```python
from build123d import *

# Parameters (mm, degrees)
SKETCH_1_R               = 5.8
SKETCH_1_R_2             = 4.55
EXTRUDE_1_DEPTH          = 2.1
SKETCH_1_3_R             = 1.7
SKETCH_1_3_R_2           = 1
EXTRUDE_2_DEPTH          = 2.9
SKETCH_1_5_R             = 5.8
SKETCH_1_5_R_2           = 4.55
SKETCH_1_5_R_3           = 1.7
SKETCH_1_5_R_4           = 1
EXTRUDE_4_DEPTH          = 0.8
SKETCH_2_R               = 5.8
SKETCH_2_R_2             = 4.75
EXTRUDE_5_DEPTH          = 4.6
EXTRUDE_6_DEPTH          = 2
CUT_EXTRUDE_1_REACH      = 11.851
FILLET_1_R               = 0.2
FILLET_2_R               = 0.3
SKETCH_6_R               = 1.15
CUT_EXTRUDE_4_DEPTH      = 0.5
CUT_EXTRUDE_5_REACH      = 16.352
CUT_EXTRUDE_5_END_RADIUS = 4.75


with BuildPart() as part:
    # Sketch 1 → Extrude 1 (new body)
    with BuildSketch(Plane.XY):
        Circle(SKETCH_1_R)
        Circle(SKETCH_1_R_2, mode=Mode.SUBTRACT)
    extrude(amount=EXTRUDE_1_DEPTH)



with BuildPart() as body_2:
    # Sketch 1_3 → Extrude 2 (new body)
    with BuildSketch(Plane.XY):
        Circle(SKETCH_1_3_R)
        Circle(SKETCH_1_3_R_2, mode=Mode.SUBTRACT)
    extrude(amount=EXTRUDE_2_DEPTH)


with BuildPart() as part_1:
    add(part.part)

    add(body_2.part)  # Extrude 4 merges body 2
    # Sketch 1_5 → Extrude 4 (add)
    with BuildSketch(Plane.XY):
        Circle(SKETCH_1_5_R)
        Circle(SKETCH_1_5_R_2, mode=Mode.SUBTRACT)
        Circle(SKETCH_1_5_R_2)
        Circle(SKETCH_1_5_R_3, mode=Mode.SUBTRACT)
        Circle(SKETCH_1_5_R_3)
        Circle(SKETCH_1_5_R_4, mode=Mode.SUBTRACT)
    extrude(amount=-EXTRUDE_4_DEPTH)

    # Sketch 2 → Extrude 5 (add)
    with BuildSketch(Plane(origin=(0, 0, -0.8), x_dir=(-1, 0, 0), z_dir=(0, 0, -1))):
        Circle(SKETCH_2_R)
        Circle(SKETCH_2_R_2, mode=Mode.SUBTRACT)
    extrude(amount=EXTRUDE_5_DEPTH)

    # Sketch 3 → Extrude 6 (add)
    with BuildSketch(Plane(origin=(0, 0, -5.4), x_dir=(-1, 0, 0), z_dir=(0, 0, -1))):
        with BuildLine():
            Line((0, 5.8), (-2.93428015, 5.8))
            ThreePointArc((-2.93428015, 5.8), (-6.5, 0), (-2.93428015, -5.8))
            Line((-2.93428015, -5.8), (0, -5.8))
            ThreePointArc((0, -5.8), (-5.8, 0), (0, 5.8))
        make_face()
        with BuildLine():
            Line((2.93428015, 5.8), (0, 5.8))
            ThreePointArc((0, 5.8), (5.8, 0), (0, -5.8))
            Line((0, -5.8), (2.93428015, -5.8))
            ThreePointArc((2.93428015, -5.8), (6.5, 0), (2.93428015, 5.8))
        make_face()
    extrude(amount=-EXTRUDE_6_DEPTH)

    # Sketch 4 → Cut-Extrude 1 (cut, up to next)
    with BuildSketch(Plane(origin=(0, 0, -0.8), x_dir=(-1, 0, 0), z_dir=(0, 0, -1)), mode=Mode.PRIVATE) as cut_extrude_1_sk1:
        with BuildLine():
            Line((-0.7, -1.549193338), (-0.7, -2.19089023))
            ThreePointArc((-0.7, -2.19089023), (0, -2.3), (0.7, -2.19089023))
            Line((0.7, -2.19089023), (0.7, -1.549193338))
            ThreePointArc((0.7, -1.549193338), (0, -1.7), (-0.7, -1.549193338))
        make_face()
    cut_extrude_1_tool1 = extrude(cut_extrude_1_sk1.sketch, amount=-CUT_EXTRUDE_1_REACH, mode=Mode.PRIVATE) & part_1.part
    # Sketch 4 → Cut-Extrude 1 (cut, up to next)
    with BuildSketch(Plane(origin=(0, 0, -0.8), x_dir=(-1, 0, 0), z_dir=(0, 0, -1)), mode=Mode.PRIVATE) as cut_extrude_1_sk2:
        with BuildLine():
            ThreePointArc((0.7, 2.19089023), (0, 2.3), (-0.7, 2.19089023))
            Line((-0.7, 2.19089023), (-0.7, 1.549193338))
            ThreePointArc((-0.7, 1.549193338), (0, 1.7), (0.7, 1.549193338))
            Line((0.7, 1.549193338), (0.7, 2.19089023))
        make_face()
    cut_extrude_1_tool2 = extrude(cut_extrude_1_sk2.sketch, amount=-CUT_EXTRUDE_1_REACH, mode=Mode.PRIVATE) & part_1.part
    # Sketch 4 → Cut-Extrude 1 (cut, up to next)
    with BuildSketch(Plane(origin=(0, 0, -0.8), x_dir=(-1, 0, 0), z_dir=(0, 0, -1)), mode=Mode.PRIVATE) as cut_extrude_1_sk3:
        with BuildLine():
            ThreePointArc((-2.19089023, 0.7), (-2.3, 0), (-2.19089023, -0.7))
            Line((-2.19089023, -0.7), (-1.549193338, -0.7))
            ThreePointArc((-1.549193338, -0.7), (-1.7, 0), (-1.549193338, 0.7))
            Line((-1.549193338, 0.7), (-2.19089023, 0.7))
        make_face()
    cut_extrude_1_tool3 = extrude(cut_extrude_1_sk3.sketch, amount=-CUT_EXTRUDE_1_REACH, mode=Mode.PRIVATE) & part_1.part
    # Sketch 4 → Cut-Extrude 1 (cut, up to next)
    with BuildSketch(Plane(origin=(0, 0, -0.8), x_dir=(-1, 0, 0), z_dir=(0, 0, -1)), mode=Mode.PRIVATE) as cut_extrude_1_sk4:
        with BuildLine():
            Line((1.549193338, -0.7), (2.19089023, -0.7))
            ThreePointArc((2.19089023, -0.7), (2.272558858, -0.354226249), (2.3, 0))
            ThreePointArc((2.3, 0), (2.272558858, 0.354226249), (2.19089023, 0.7))
            Line((2.19089023, 0.7), (1.549193338, 0.7))
            ThreePointArc((1.549193338, 0.7), (1.661870734, 0.358030253), (1.7, 0))
            ThreePointArc((1.7, 0), (1.661870734, -0.358030253), (1.549193338, -0.7))
        make_face()
    cut_extrude_1_tool4 = extrude(cut_extrude_1_sk4.sketch, amount=-CUT_EXTRUDE_1_REACH, mode=Mode.PRIVATE) & part_1.part
    # Sketch 4 → Cut-Extrude 1 (cut, up to next)
    with BuildSketch(Plane(origin=(0, 0, -0.8), x_dir=(-1, 0, 0), z_dir=(0, 0, -1)), mode=Mode.PRIVATE) as cut_extrude_1_sk5:
        with BuildLine():
            Line((-0.7, -1.549193338), (-0.7, -2.19089023))
            ThreePointArc((-0.7, -2.19089023), (0, -2.3), (0.7, -2.19089023))
            Line((0.7, -2.19089023), (0.7, -1.549193338))
            ThreePointArc((0.7, -1.549193338), (0, -1.7), (-0.7, -1.549193338))
        make_face()
    cut_extrude_1_tool5 = extrude(cut_extrude_1_sk5.sketch, amount=-CUT_EXTRUDE_1_REACH, mode=Mode.PRIVATE) & part_1.part
    # Sketch 4 → Cut-Extrude 1 (cut, up to next)
    with BuildSketch(Plane(origin=(0, 0, -0.8), x_dir=(-1, 0, 0), z_dir=(0, 0, -1)), mode=Mode.PRIVATE) as cut_extrude_1_sk6:
        with BuildLine():
            ThreePointArc((0.7, 2.19089023), (0, 2.3), (-0.7, 2.19089023))
            Line((-0.7, 2.19089023), (-0.7, 1.549193338))
            ThreePointArc((-0.7, 1.549193338), (0, 1.7), (0.7, 1.549193338))
            Line((0.7, 1.549193338), (0.7, 2.19089023))
        make_face()
    cut_extrude_1_tool6 = extrude(cut_extrude_1_sk6.sketch, amount=-CUT_EXTRUDE_1_REACH, mode=Mode.PRIVATE) & part_1.part
    # Sketch 4 → Cut-Extrude 1 (cut, up to next)
    with BuildSketch(Plane(origin=(0, 0, -0.8), x_dir=(-1, 0, 0), z_dir=(0, 0, -1)), mode=Mode.PRIVATE) as cut_extrude_1_sk7:
        with BuildLine():
            ThreePointArc((-2.19089023, 0.7), (-2.3, 0), (-2.19089023, -0.7))
            Line((-2.19089023, -0.7), (-1.549193338, -0.7))
            ThreePointArc((-1.549193338, -0.7), (-1.7, 0), (-1.549193338, 0.7))
            Line((-1.549193338, 0.7), (-2.19089023, 0.7))
        make_face()
    cut_extrude_1_tool7 = extrude(cut_extrude_1_sk7.sketch, amount=-CUT_EXTRUDE_1_REACH, mode=Mode.PRIVATE) & part_1.part
    # Sketch 4 → Cut-Extrude 1 (cut, up to next)
    with BuildSketch(Plane(origin=(0, 0, -0.8), x_dir=(-1, 0, 0), z_dir=(0, 0, -1)), mode=Mode.PRIVATE) as cut_extrude_1_sk8:
        with BuildLine():
            Line((1.549193338, -0.7), (2.19089023, -0.7))
            ThreePointArc((2.19089023, -0.7), (2.272558858, -0.354226249), (2.3, 0))
            ThreePointArc((2.3, 0), (2.272558858, 0.354226249), (2.19089023, 0.7))
            Line((2.19089023, 0.7), (1.549193338, 0.7))
            ThreePointArc((1.549193338, 0.7), (1.661870734, 0.358030253), (1.7, 0))
            ThreePointArc((1.7, 0), (1.661870734, -0.358030253), (1.549193338, -0.7))
        make_face()
    cut_extrude_1_tool8 = extrude(cut_extrude_1_sk8.sketch, amount=-CUT_EXTRUDE_1_REACH, mode=Mode.PRIVATE) & part_1.part
    add(cut_extrude_1_tool1.solids().sort_by_distance((0, -1.956551, -0.8))[0], mode=Mode.SUBTRACT)
    add(cut_extrude_1_tool2.solids().sort_by_distance((0, 1.956551, -0.8))[0], mode=Mode.SUBTRACT)
    add(cut_extrude_1_tool3.solids().sort_by_distance((1.956551, 0, -0.8))[0], mode=Mode.SUBTRACT)
    add(cut_extrude_1_tool4.solids().sort_by_distance((-1.956551, 0, -0.8))[0], mode=Mode.SUBTRACT)
    add(cut_extrude_1_tool5.solids().sort_by_distance((0, -1.956551, -0.8))[0], mode=Mode.SUBTRACT)
    add(cut_extrude_1_tool6.solids().sort_by_distance((0, 1.956551, -0.8))[0], mode=Mode.SUBTRACT)
    add(cut_extrude_1_tool7.solids().sort_by_distance((1.956551, 0, -0.8))[0], mode=Mode.SUBTRACT)
    add(cut_extrude_1_tool8.solids().sort_by_distance((-1.956551, 0, -0.8))[0], mode=Mode.SUBTRACT)

    # Fillet 1
    fillet_1_edges = [part_1.edges().sort_by_distance(p)[0] for p in [
        (-1.7, 0, 2.9),
    ]]
    fillet(fillet_1_edges, radius=FILLET_1_R)

    # Fillet 2
    fillet_2_edges = [part_1.edges().sort_by_distance(p)[0] for p in [
        (4.75, 0, -5.4),
    ]]
    fillet(fillet_2_edges, radius=FILLET_2_R)

    # Sketch 6 → Cut-Extrude 4 (cut)
    with BuildSketch(Plane(origin=(0, 0, -0.8), x_dir=(-1, 0, 0), z_dir=(0, 0, -1))):
        Circle(SKETCH_6_R)
    extrude(amount=-CUT_EXTRUDE_4_DEPTH, mode=Mode.SUBTRACT)

    # Cut-Extrude 5: up to this cylinder (the profile starts outside it)
    cut_extrude_5_end = Plane(origin=(0, 0, -4.843393), z_dir=(0, 0, 1)) * Cylinder(CUT_EXTRUDE_5_END_RADIUS, 44.284964, mode=Mode.PRIVATE)
    # Sketch 7 → Cut-Extrude 5 (cut, up to the surface)
    with BuildSketch(Plane(origin=(0, 5.8, 0), x_dir=(1, 0, 0), z_dir=(0, 1, 0)), mode=Mode.PRIVATE) as cut_extrude_5_sk1:
        with BuildLine():
            Line((-0.7, 5.4), (-0.7, 4.6))
            ThreePointArc((-0.7, 4.6), (0, 5.3), (0.7, 4.6))
            Line((0.7, 4.6), (0.7, 5.4))
            Line((0.7, 5.4), (-0.7, 5.4))
        make_face()
    cut_extrude_5_tool1 = extrude(cut_extrude_5_sk1.sketch, amount=-CUT_EXTRUDE_5_REACH, mode=Mode.PRIVATE) - cut_extrude_5_end
    add(cut_extrude_5_tool1.solids().sort_by_distance((0, 5.8, -5.383875))[0], mode=Mode.SUBTRACT)
    # Sketch 7 → Cut-Extrude 5 (cut, up to the surface)
    with BuildSketch(Plane(origin=(0, 5.8, 0), x_dir=(1, 0, 0), z_dir=(0, 1, 0)), mode=Mode.PRIVATE) as cut_extrude_5_sk2:
        with BuildLine():
            ThreePointArc((0.7, 4.6), (0, 5.3), (-0.7, 4.6))
            Line((-0.7, 4.6), (0.7, 4.6))
        make_face()
    cut_extrude_5_tool2 = extrude(cut_extrude_5_sk2.sketch, amount=-CUT_EXTRUDE_5_REACH, mode=Mode.PRIVATE) - cut_extrude_5_end
    add(cut_extrude_5_tool2.solids().sort_by_distance((0, 5.8, -4.897089))[0], mode=Mode.SUBTRACT)
    # Sketch 7 → Cut-Extrude 5 (cut, up to the surface)
    with BuildSketch(Plane(origin=(0, 5.8, 0), x_dir=(1, 0, 0), z_dir=(0, 1, 0)), mode=Mode.PRIVATE) as cut_extrude_5_sk3:
        with BuildLine():
            Line((0.7, 4.6), (-0.7, 4.6))
            ThreePointArc((-0.7, 4.6), (0, 3.9), (0.7, 4.6))
        make_face()
    cut_extrude_5_tool3 = extrude(cut_extrude_5_sk3.sketch, amount=-CUT_EXTRUDE_5_REACH, mode=Mode.PRIVATE) - cut_extrude_5_end
    add(cut_extrude_5_tool3.solids().sort_by_distance((0, 5.8, -4.302911))[0], mode=Mode.SUBTRACT)
    # Sketch 7 → Cut-Extrude 5 (cut, up to the surface)
    with BuildSketch(Plane(origin=(0, 5.8, 0), x_dir=(1, 0, 0), z_dir=(0, 1, 0)), mode=Mode.PRIVATE) as cut_extrude_5_sk4:
        with BuildLine():
            ThreePointArc((0.7, 4.6), (0, 5.3), (-0.7, 4.6))
            Line((-0.7, 4.6), (0.7, 4.6))
        make_face()
    cut_extrude_5_tool4 = extrude(cut_extrude_5_sk4.sketch, amount=-CUT_EXTRUDE_5_REACH, mode=Mode.PRIVATE) - cut_extrude_5_end
    add(cut_extrude_5_tool4.solids().sort_by_distance((0, 5.8, -4.897089))[0], mode=Mode.SUBTRACT)
    # Sketch 7 → Cut-Extrude 5 (cut, up to the surface)
    with BuildSketch(Plane(origin=(0, 5.8, 0), x_dir=(1, 0, 0), z_dir=(0, 1, 0)), mode=Mode.PRIVATE) as cut_extrude_5_sk5:
        with BuildLine():
            Line((0.7, 4.6), (-0.7, 4.6))
            ThreePointArc((-0.7, 4.6), (0, 3.9), (0.7, 4.6))
        make_face()
    cut_extrude_5_tool5 = extrude(cut_extrude_5_sk5.sketch, amount=-CUT_EXTRUDE_5_REACH, mode=Mode.PRIVATE) - cut_extrude_5_end
    add(cut_extrude_5_tool5.solids().sort_by_distance((0, 5.8, -4.302911))[0], mode=Mode.SUBTRACT)


solid = part_1.part
```
Verification items for the finished model (mm, model axes). A direction names the side the tool comes from. Coordinates: 2 decimals unless noted, no trailing zeros. Loops run counter-clockwise (first coordinate to the right, second up) from the corner with the lowest first, then second, coordinate; pieces in that order, holes last. Notation, with made-up numbers: (52.5, 47.25) - (96.5, 47.25) arc R22 ccw to (96.5, 84.25) - close; hole circle Ø11 at (-21.5, -1.75). An arc over 180 degrees is marked (long way). Return JSON: item names as keys, results as strings.
1. Section check B-B, the plane z = -2. Record the boundary of the cut face in (x, y).
Established:
{"outline": "circle Ø11.6 at (0, 0); hole circle Ø9.5 at (0, 0)"}
2. Thickness scan on L1, parallel to Y at x = 0, z = 1.9; L2, parallel to X at y = 0, z = -1.75; L3, parallel to Y at x = 0, z = -0.6. Record the ranges inside material, lowest first.
Established:
{"L1": "y = -5.8 to -4.55, -1.7 to -1, 1 to 1.7, 4.55 to 5.8", "L2": "x = -5.8 to -4.75, 4.75 to 5.8", "L3": "y = -5.8 to -2.3, -1.7 to -1.15, 1.15 to 1.7, 2.3 to 5.8"}
3. Mould release check, pull along Y, two halves, no side actions. Record for faces 4 (the flat face through (-0.7, 5, -5)), 5 (the flat face through (0, 5.8, -3.7)), 6 (the cylindrical face through (0.91, -0.7, -0.55)): +Y half, -Y half, draft (parallel to the pull), parting line (faces both ways), or undercut.
Established:
{"face 4": "draft", "face 5": "+Y half", "face 6": "undercut"}
4. Go/stop test with flat-tipped pins: pin 1 (5.5 mm diameter, centred on x = 0, y = 0, fed in from -Z); pin 2 (0.7 mm diameter, centred on y = -2, z = -0.5, fed in from +X); pin 3 (0.7 mm diameter, centred on x = -2, z = -0.5, fed in from -Y); pin 4 (1.8 mm diameter, centred on x = 0, y = 0, fed in from +Z). Record where each tip stops, or that it passes through.
Established:
{"pin 1": "stops at z = -0.8", "pin 2": "stops at x = 5.56", "pin 3": "stops at y = -5.56", "pin 4": "passes through"}
5. Tool access check on faces 1 (the flat face through (6, 0, -3.4)), 2 (the cylindrical face through (0, 5.3, -3.9)), 3 (the flat face through (1, -2, 0)). Record the directions out of +Z, -Z, +X, -X, +Y, -Y that give a thin tool (end or side, any length) a straight path to the whole face; none if there is none.
Established:
{"face 1": "+Z, +X", "face 2": "-Z, +Y", "face 3": "+Z"}
6. Section check A-A, the plane z = 1. Record the boundary of the cut face in (x, y), then the cut area to 3 significant figures.
Established:
{"outline": "circle Ø11.6 at (0, 0); circle Ø3.4 at (0, 0); hole circle Ø9.1 at (0, 0); hole circle Ø2 at (0, 0)", "area": "46.6 mm2"}
